Read the model definition and answer for the solid it produces. Units are mm, in the model's axes. A direction names the side the tool comes from. Give positions to 0.01 mm unless a question says otherwise; leave off trailing zeros. Loops run counter-clockwise (first coordinate to the right, second up) from the corner with the lowest first, then second, coordinate; pieces in that order, holes last. Notation, with made-up numbers: (-1, 69) - (14, 69) arc R7 cw to (14, 79) - close; hole circle Ø1 at (71, 19.5). An arc over 180 degrees is marked (long way). Write item = value, one per line. Start each with the question number.
from build123d import *

# Parameters (mm, degrees)
SKETCH1_W            = 78
SKETCH1_H            = 78
BOSS_EXTRUDE1_DEPTH  = 2
SKETCH2_W            = 30
SKETCH2_H            = 30
BOSS_EXTRUDE2_DEPTH  = 60
SKETCH3_W            = 26
SKETCH3_H            = 26
CUT_EXTRUDE1_DEPTH   = 62
SKETCH4_W            = 28
SKETCH4_H            = 2.5
CUT_EXTRUDE2_DEPTH   = 28
SKETCH5_W            = 26
SKETCH5_H            = 10
CUT_EXTRUDE3_DEPTH   = 2
SKETCH6_W            = 28
SKETCH6_H            = 2.5
CUT_EXTRUDE4_DEPTH   = 1
SKETCH7_W            = 28
SKETCH7_H            = 2.5
CUT_EXTRUDE5_DEPTH   = 1
SKETCH14_R           = 1.75
BOSS_EXTRUDE8_DEPTH  = 5
SKETCH16_W           = 4
SKETCH16_H           = 5
BOSS_EXTRUDE10_DEPTH = 2
SKETCH17_W           = 2
SKETCH17_H           = 10
BOSS_EXTRUDE11_DEPTH = 5
SKETCH18_W           = 10
SKETCH18_H           = 2
BOSS_EXTRUDE12_DEPTH = 3
SKETCH21_W           = 78
SKETCH21_H           = 78
BOSS_EXTRUDE13_DEPTH = 53
SKETCH15_W           = 43
SKETCH15_H           = 43
CUT_EXTRUDE6_DEPTH   = 53
SKETCH23_W           = 5
SKETCH23_H           = 2
BOSS_EXTRUDE15_DEPTH = 5
SKETCH24_W           = 26
SKETCH24_H           = 26
CUT_EXTRUDE9_DEPTH   = 51
SKETCH27_W           = 26
SKETCH27_H           = 26
CUT_EXTRUDE10_DEPTH  = 2
BOSS_EXTRUDE16_DEPTH = 26
SKETCH31_W           = 13
SKETCH31_H           = 13
CUT_EXTRUDE12_DEPTH  = 10
SKETCH32_R           = 2
CUT_EXTRUDE13_DEPTH  = 2
SKETCH33_R           = 2
CUT_EXTRUDE14_DEPTH  = 2
SKETCH36_R           = 1.75
BOSS_EXTRUDE17_DEPTH = 4


with BuildPart() as part:
    # Sketch1 → Boss-Extrude1 (new body)
    with BuildSketch(Plane(origin=(0, 0, 0), x_dir=(1, 0, 0), z_dir=(0, 1, 0))):
        Rectangle(SKETCH1_W, SKETCH1_H)
    extrude(amount=BOSS_EXTRUDE1_DEPTH)

    # Sketch2 → Boss-Extrude2 (add)
    with BuildSketch(Plane(origin=(0, 2, 0), x_dir=(1, 0, 0), z_dir=(0, 1, 0))):
        with Locations((24, 24)):
            Rectangle(SKETCH2_W, SKETCH2_H)
    extrude(amount=BOSS_EXTRUDE2_DEPTH)

    # Sketch3 → Cut-Extrude1 (cut)
    with BuildSketch(Plane(origin=(0, 62, 0), x_dir=(1, 0, 0), z_dir=(0, 1, 0))):
        with Locations((24, 24)):
            Rectangle(SKETCH3_W, SKETCH3_H)
    extrude(amount=-CUT_EXTRUDE1_DEPTH, mode=Mode.SUBTRACT)

    # Sketch4 → Cut-Extrude2 (cut)
    with BuildSketch(Plane.ZY.offset(-9)):
        with Locations((-23.934548619, 3.25)):
            Rectangle(SKETCH4_W, SKETCH4_H)
    extrude(amount=-CUT_EXTRUDE2_DEPTH, mode=Mode.SUBTRACT)

    # Sketch5 → Cut-Extrude3 (cut)
    with BuildSketch(Plane.XY.offset(-9)):
        with Locations((24, 9)):
            Rectangle(SKETCH5_W, SKETCH5_H)
    extrude(amount=-CUT_EXTRUDE3_DEPTH, mode=Mode.SUBTRACT)

    # Sketch6 → Cut-Extrude4 (cut)
    with BuildSketch(Plane.ZY.offset(-37)):
        with Locations((-23, 7.5)):
            Rectangle(SKETCH6_W, SKETCH6_H)
    extrude(amount=-CUT_EXTRUDE4_DEPTH, mode=Mode.SUBTRACT)

    # Sketch7 → Cut-Extrude5 (cut)
    with BuildSketch(Plane(origin=(11, 0, 0), x_dir=(0, 0, -1), z_dir=(1, 0, 0))):
        with Locations((23, 7.5)):
            Rectangle(SKETCH7_W, SKETCH7_H)
    extrude(amount=-CUT_EXTRUDE5_DEPTH, mode=Mode.SUBTRACT)

    # Sketch14 → Boss-Extrude8 (add)
    with BuildSketch(Plane(origin=(0, 2, 0), x_dir=(1, 0, 0), z_dir=(0, 1, 0))):
        with Locations((-3.25, -24.64)):
            Circle(SKETCH14_R)
    extrude(amount=BOSS_EXTRUDE8_DEPTH)

    # Sketch16 → Boss-Extrude10 (add)
    with BuildSketch(Plane(origin=(0, 2, 0), x_dir=(1, 0, 0), z_dir=(0, 1, 0))):
        with Locations((22, -22.14)):
            Rectangle(SKETCH16_W, SKETCH16_H)
        with Locations((22, -27.14)):
            Rectangle(SKETCH16_W, SKETCH16_H)
    extrude(amount=BOSS_EXTRUDE10_DEPTH)

    # Sketch17 → Boss-Extrude11 (add)
    with BuildSketch(Plane(origin=(0, 2, 0), x_dir=(1, 0, 0), z_dir=(0, 1, 0))):
        with Locations((25, -24.64)):
            Rectangle(SKETCH17_W, SKETCH17_H)
    extrude(amount=BOSS_EXTRUDE11_DEPTH)

    # Sketch18 → Boss-Extrude12 (add)
    with BuildSketch(Plane(origin=(0, 2, 0), x_dir=(1, 0, 0), z_dir=(0, 1, 0))):
        with Locations((-24.64, 25)):
            Rectangle(SKETCH18_W, SKETCH18_H)
    extrude(amount=BOSS_EXTRUDE12_DEPTH)

    # Sketch21 → Boss-Extrude13 (add)
    with BuildSketch(Plane.XZ):
        Rectangle(SKETCH21_W, SKETCH21_H)
    extrude(amount=BOSS_EXTRUDE13_DEPTH)

    # Sketch15 → Cut-Extrude6 (cut)
    with BuildSketch(Plane(origin=(0, 2, 0), x_dir=(1, 0, 0), z_dir=(0, 1, 0))):
        with Locations((-24.64, -3.25)):
            Rectangle(SKETCH15_W, SKETCH15_H)
    extrude(amount=-CUT_EXTRUDE6_DEPTH, mode=Mode.SUBTRACT)

    # Sketch23 → Boss-Extrude15 (add)
    with BuildSketch(Plane.ZY.offset(3.14)):
        with Locations((22.25, 1)):
            Rectangle(SKETCH23_W, SKETCH23_H)
    extrude(amount=BOSS_EXTRUDE15_DEPTH)

    # Sketch24 → Cut-Extrude9 (cut)
    with BuildSketch(Plane(origin=(0, 0, 0), x_dir=(1, 0, 0), z_dir=(0, 1, 0))):
        with Locations((24, 24)):
            Rectangle(SKETCH24_W, SKETCH24_H)
    extrude(amount=-CUT_EXTRUDE9_DEPTH, mode=Mode.SUBTRACT)

    # Sketch27 → Cut-Extrude10 (cut)
    with BuildSketch(Plane(origin=(0, 0, -39), x_dir=(-1, 0, 0), z_dir=(0, 0, -1))):
        with Locations((-24, -38)):
            Rectangle(SKETCH27_W, SKETCH27_H)
    extrude(amount=-CUT_EXTRUDE10_DEPTH, mode=Mode.SUBTRACT)

    # Sketch28 → Boss-Extrude16 (add)
    with BuildSketch(Plane(origin=(11, 0, 0), x_dir=(0, 0, -1), z_dir=(1, 0, 0))):
        Polygon((39, -51), (11, -51), (11, -24.5), align=None)
    extrude(amount=BOSS_EXTRUDE16_DEPTH)

    # Sketch31 → Cut-Extrude12 (cut)
    with BuildSketch(Plane(origin=(0, 2, 0), x_dir=(1, 0, 0), z_dir=(0, 1, 0))):
        with Locations((2.5, 32.5)):
            Rectangle(SKETCH31_W, SKETCH31_H)
    extrude(amount=-CUT_EXTRUDE12_DEPTH, mode=Mode.SUBTRACT)

    # Sketch32 → Cut-Extrude13 (cut)
    with BuildSketch(Plane(origin=(39, 0, 0), x_dir=(0, 0, -1), z_dir=(1, 0, 0))):
        with Locations((34, -3)):
            Circle(SKETCH32_R)
    extrude(amount=-CUT_EXTRUDE13_DEPTH, mode=Mode.SUBTRACT)

    # Sketch33 → Cut-Extrude14 (cut)
    with BuildSketch(Plane(origin=(11, 0, 0), x_dir=(0, 0, -1), z_dir=(1, 0, 0))):
        with Locations((34, -3)):
            Circle(SKETCH33_R)
    extrude(amount=-CUT_EXTRUDE14_DEPTH, mode=Mode.SUBTRACT)

    # Sketch36 → Boss-Extrude17 (add)
    with BuildSketch(Plane(origin=(0, 7, 0), x_dir=(1, 0, 0), z_dir=(0, 1, 0))):
        with Locations((-3.25, -24.64)):
            Circle(SKETCH36_R)
    extrude(amount=BOSS_EXTRUDE17_DEPTH)


solid = part.part
1. A tool of negligible diameter and unlimited length cuts with its end or side. For faces 5 (the flat face through (26, 4, 25)), 6 (the flat face through (-25, 3, -26)), 7 (the cylindrical face through (-4.64, 6.44, 25.7)), 8 (the flat face through (-4, -3, -32)), 9 (the flat face through (22, 4, 25)), from which of +Z, -Z, +X, -X, +Y, -Y can it reach the whole face along a straight path? Write none if from no direction.
2. A cutting plane is placed at D-D on y = -3. Give the vertices of the cut face in (x, z).
3. Given P1, Ø1.6, axis at y = 3.5, z = -24.5, coming from the -X side; P2, Ø24, axis at x = 26.5, y = 31, coming from the +Z side; P3, Ø1.6, axis at y = 3.5, z = 23, coming from the -X side; P4, Ø14.5, axis at x = 4, z = -30.5, coming from the +Y side, each flat-ended and moving along its own axis, determine where each tip first touches the part or whether it passes through.
4. A cutting plane is placed at C-C on z = -34. Give the number of separate pieces and of enclosed holes in the cut face, and give its area (3 significant figures).
5. A cutting plane is placed at A-A on x = 14. Give the vertices of the cut face in (y, z).
6. For a pull along Y with two mould halves and no side action, classify faces 1 (the flat face through (17, -7, -39)), 2 (the flat face through (2, -8, -33)), 3 (the flat face through (10, 4.5, -28)), 4 (the flat face through (23, 3, -9.935)) as released by +Y, released by -Y, zero draft, split by the parting line, or undercut.
7. Consider line 1 along Y through (x, z) = (37.75, -34); line 2 along X through (y, z) = (39.5, -25); line 3 along Z through (x, y) = (17, 39). Determine where each line is inside the solid, lowest interval first. Write a range as [from, to].
8. A cutting plane is placed at B-B on y = 21.5. Give the vertices of the cut face in (x, z).
Reply:
q1.face_5 = +Z, +X, +Y
q1.face_6 = -Z, -X, +Y
q1.face_7 = +Y
q1.face_8 = -Z, +Y
q1.face_9 = +Z, +Y
q2.outline = (-39, -39) - (-4, -39) - (-4, -26) - (9, -26) - (9, -32) - (11, -32) - (11, -11) - (37, -11) - (37, -32) - (39, -32) - (39, 39) - (-39, 39) - (-39, 24.75) - (-3.14, 24.75) - (-3.14, -18.25) - (-39, -18.25) - close; (9, -39) - (39, -39) - (39, -36) - (37, -36) - (37, -37) - (11, -37) - (11, -36) - (9, -36) - close
q3.P1 = -29.64
q3.P2 = -9
q3.P3 = -4.79
q3.P4 = 62
q4.separate_pieces = 4
q4.enclosed_holes = 0
q4.area = 3,120 mm^2
q5.outline = (-53, -39) - (-51, -39) - (-24.5, -11) - (2, -11) - (2, -9.93) - (4, -9.93) - (4, -9) - (2, -9) - (2, 39) - (-53, 39) - close; (-25, -39) - (62, -39) - (62, -37) - (4.5, -37) - (4.5, -37.93) - (2, -37.93) - (2, -37) - (-25, -37) - close; (14, -11) - (62, -11) - (62, -9) - (14, -9) - close
q6.face_1 = zero draft
q6.face_2 = released by +Y
q6.face_3 = undercut
q6.face_4 = undercut
q7.line_1 = [-53, -5], [-1, 6.25], [8.75, 62]
q7.line_2 = [9, 11], [37, 39]
q7.line_3 = [-39, -37], [-11, -9]
q8.outline = (9, -39) - (39, -39) - (39, -9) - (9, -9) - close; hole (11, -37) - (37, -37) - (37, -11) - (11, -11) - close
